Build history of the part. All positions in model axes, mm. Round coordinates to 2 decimals unless told otherwise and drop trailing zeros. Order: outer loops, then holes, each group sorted by start corner. A loop starts at its lowest first (then second) coordinate and runs counter-clockwise, first axis right, second up. Notation, with made-up numbers: (58.25, 69) - (76.25, 69) arc R21 ccw to (76.25, 79) - close; hole circle Ø5 at (61, -29). An arc over 180 degrees is marked (long way). One line per question, with ' | ' between items. Start each with the question number.
from build123d import *

# Parameters (mm, degrees)
SALIENTE_EXTRUIR3_DEPTH = 15


with BuildPart() as part:
    # Croquis2 → Saliente-Extruir3 (new body)
    with BuildSketch(Plane(origin=(0, 0, 0), x_dir=(0, 0, -1), z_dir=(1, 0, 0))):
        with BuildLine():
            Line((0, 0), (375, 0))
            Line((375, 0), (375, 50))
            Line((375, 50), (351, 50))
            Line((351, 50), (351, 46.5))
            ThreePointArc((351, 46.5), (347, 42.5), (343, 46.5))
            Line((343, 46.5), (343, 50))
            Line((343, 50), (325, 50))
            Line((325, 50), (325, 15))
            Line((325, 15), (50, 15))
            Line((50, 15), (50, 50))
            Line((50, 50), (32, 50))
            Line((32, 50), (32, 46.5))
            ThreePointArc((32, 46.5), (28, 42.5), (24, 46.5))
            Line((24, 46.5), (24, 50))
            Line((24, 50), (0, 50))
            Line((0, 50), (0, 0))
        make_face()
    extrude(amount=SALIENTE_EXTRUIR3_DEPTH)


solid = part.part
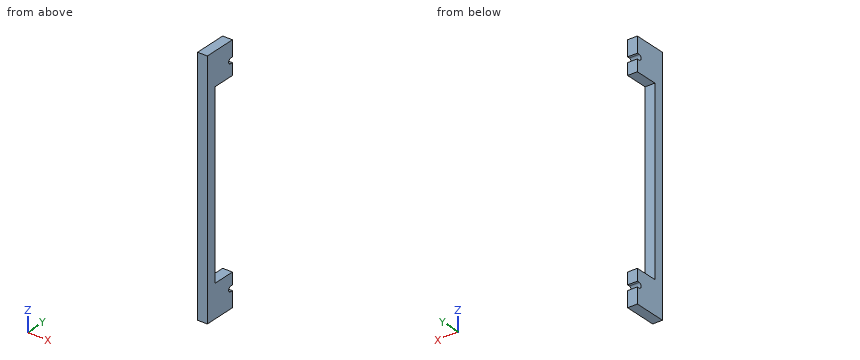
Item 1: Slice it at B-B (x = 4). Write the cut outline in (y, z), plus the area to 3 significant figures.
Item 2: Slice it at D-D (z = -142). Write the cut outline in (x, y), plus the area to 3 significant figures.
Item 3: Slice it at C-C (z = -347). Write the cut outline in (x, y), plus the area to 4 significant figures.
Item 4: Pin check, flat tip, straight feed: pin 1 (4 mm diameter, centred on x = 9.5, z = -270, fed in from +Y). Stop position of the tip, or through.
Item 5: Wall check: line 1 along Z through (x, y) = (2.75, 46); line 2 along Z through (x, y) = (3.25, 43); line 3 along Z through (x, y) = (14.25, 25.5). Give the ranges that are in metal, low to high. Write a range as [from, to].
Item 6: Slice it at A-A (y = 35.5). Write the cut outline in (x, z).
A:
1) outline: (0, -375) - (50, -375) - (50, -351) - (46.5, -351) arc R4 cw to (46.5, -343) - (50, -343) - (50, -325) - (15, -325) - (15, -50) - (50, -50) - (50, -32) - (46.5, -32) arc R4 cw to (46.5, -24) - (50, -24) - (50, 0) - (0, 0) - close | area: 9,020 mm^2
2) outline: (0, 0) - (15, 0) - (15, 15) - (0, 15) - close | area: 225 mm^2
3) outline: (0, 0) - (15, 0) - (15, 42.5) - (0, 42.5) - close | area: 637.5 mm^2
4) pin 1: y = 15
5) line 1: [-375, -350.97], [-343.03, -325], [-50, -31.97], [-24.03, 0] | line 2: [-375, -348.94], [-345.06, -325], [-50, -29.94], [-26.06, 0] | line 3: [-375, -325], [-50, 0]
6) outline: (0, -375) - (15, -375) - (15, -325) - (0, -325) - close; (0, -50) - (15, -50) - (15, 0) - (0, 0) - close
